Geometry: final body of the model. Coordinates: model frame, mm. A direction names the side the tool comes from. Give positions to 0.01 mm unless a question says otherwise; leave off trailing zeros. Order: outer loops, then holes, each group sorted by start corner. A loop starts at its lowest first (then second) coordinate and runs counter-clockwise, first axis right, second up. Notation, with made-up numbers: (-35, -31) -> (-23, -31) arc R10 cw to (-23, -24) -> close; hole circle Ø8 at (-31.75, 75). An arc over 180 degrees is marked (long way). Write item = value, one per line.
Solid Edge part; units mm, degrees
sketch "Sketch1" plane through (0, 0, 0) normal (0, -1, 0) x (1, 0, 0)
  line L0 (-60, 37) -> (-15, 0)
  line L1 (-15, 0) -> (15, 0)
  line L2 (15, 0) -> (60, 37)
  line L3 (60, 37) -> (-60, 37)
  dimension "D1" = 15
  dimension "D2" = 60
  dimension "D3" = 60
extrude "Protrusion1" add sketch "Sketch1" against normal blind 40
sketch "Sketch2" plane through (0, 40, 18.5) normal (0, 1, 0) x (-1, 0, 0)
  line L0 (-8, -18.5) -> (8, -18.5)
  line L1 (8, -18.5) -> (8, 11.5)
  line L2 (8, 11.5) -> (-8, 11.5)
  line L3 (-8, 11.5) -> (-8, -18.5)
  line L4 (-40.4647, 11.5) -> (-15, -9.4376)
  line L5 (-15, -9.4376) -> (-15, 11.5)
  line L6 (-15, 11.5) -> (-40.4647, 11.5)
  line L7 (40.4647, 11.5) -> (15, -9.4376)
  line L8 (15, -9.4376) -> (15, 11.5)
  line L9 (15, 11.5) -> (40.4647, 11.5)
  dimension "D1" = 8
extrude "ExtrudedCutout_1" cut sketch "Sketch2" against normal blind 33
sketch "Sketch3" plane through (0, 7, 15) normal (0, 1, 0) x (-1, 0, 0)
  circle A0 centre (0, -11.5) radius 1.7
  circle A1 centre (0, 4.5) radius 1.7
extrude "Cutout1" cut sketch "Sketch3" against normal through all
sketch "Sketch4" plane through (0, 0, 0) normal (1, 0, 0) x (0, 1, 0)
  line L0 (7, 0) -> (40, 30)
extrude "Cutout2" cut sketch "Sketch4" against normal through all and the other way through all material side at (0, 23.5336, 14.963)
sketch "Sketch5" plane through (0, 0, 0) normal (1, 0, 0) x (0, 1, 0)
  line L0 (40, 37) -> (40, 58)
  line L1 (40, 58) -> (33, 58)
  line L2 (33, 58) -> (33, 40)
  arc A0 (30, 37) -> (33, 40) centre (30, 40) ccw
  line L3 (40, 37) -> (30, 37)
  dimension "D1" = 40
  dimension "D2" = 40
extrude "ExtrudedProtrusion_3" add sketch "Sketch5" along normal mid plane 120
fillet "Round_1" radius 3 1 edges at (0, 0, 37)
extrude "Cutout3" [suppressed]
sketch "Sketch6" plane through (0, 33, 49) normal (0, -1, 0) x (1, 0, 0)
  line L0 (-50, 1.7) -> (50, 1.7)
  arc A0 (50, 1.7) -> (50, -1.7) centre (50, 0) cw
  line L1 (50, -1.7) -> (-50, -1.7)
  arc A1 (-50, 1.7) -> (-50, -1.7) centre (-50, 0) ccw
  dimension "D1" = 50
extrude "ExtrudedProtrusion_4" add sketch "Sketch6" along normal blind 25
properties material "ABS Plastic, medium impact"
1) Section query B-B (y = 13). Output: boundary loops of the cut face in (x, z).
Check sheet entries:
outline = (-60, 37) -> (-21.63, 5.45) -> (-8, 5.45) -> (-8, 30) -> (8, 30) -> (8, 5.45) -> (21.63, 5.45) -> (60, 37) -> close; (-50, 47.3) -> (50, 47.3) arc R1.7 ccw to (50, 50.7) -> (-50, 50.7) arc R1.7 ccw to start; hole (-40.46, 30) -> (-15, 9.06) -> (-15, 30) -> close; hole (15, 9.06) -> (40.46, 30) -> (15, 30) -> close
2) First-contact query: P1, Ø24, axis at y = 18.5, z = 10, coming from the -X side; P2, Ø6.5, axis at y = 24, z = 22.5, coming from the -X side; P3, Ø5.5, axis at x = -25.5, z = 48.5, coming from the -Y side; P4, Ø4, axis at x = 0, z = 3.5, coming from the -Y side. Flat tips, straight axial feed; report the tip coordinate or a pass-through.
Check sheet entries:
P1 = -41.76
P2 = -46.32
P3 = 8
P4 = 0
3) Mould query, pull axis X, two halves, no side actions, for faces 4 (the face through (1, 8, 49)), 5 (the face through (-51.7, 20.7, 49)), 6 (the face through (-15, 20, 22)). Classes: +X half, -X half, draft (parallel to the pull), parting line (faces both ways), or undercut.
Check sheet entries:
face_4 = draft
face_5 = -X half
face_6 = undercut
4) Section query A-A (x = 0). Output: boundary loops of the cut face in (y, z), plus the area to 3 significant figures.
Check sheet entries:
outline = (0, 0) -> (7, 0) -> (7, 1.8) -> (0, 1.8) -> close; (0, 5.2) -> (7, 5.2) -> (7, 17.8) -> (0, 17.8) -> close; (0, 21.2) -> (7, 21.2) -> (7, 30) -> (40, 30) -> (40, 58) -> (33, 58) -> (33, 50.7) -> (8, 50.7) -> (8, 47.3) -> (33, 47.3) -> (33, 40) arc R3 cw to (30, 37) -> (3, 37) arc R3 ccw to (0, 34) -> close
area = 674 mm²
5) Line query: line 1 (Z direction, x = 0, y = 5.25); line 2 (Z direction, x = 0, y = 1.5); line 3 (X direction, y = 12, z = 6.5). Output: solid intervals per line, ascending. Write a range as from..to.
Check sheet entries:
line_1 = 0..1.8, 5.2..17.8, 21.2..37
line_2 = 0..1.8, 5.2..17.8, 21.2..36.6
line_3 = -22.91..-8, 8..22.91
6) Section query C-C (z = 49). Output: boundary loops of the cut face in (x, y).
Check sheet entries:
outline = (-60, 33) -> (-51.7, 33) -> (-51.7, 8) -> (51.7, 8) -> (51.7, 33) -> (60, 33) -> (60, 40) -> (-60, 40) -> close
7) Reachability of faces 1 (the face through (-1, 21, 50.7)), 2 (the face through (8, 16, 22)), 3 (the face through (22, 7, 24)) from +Z, -Z, +X, -X, +Y, -Y: full face, straight path, thin tool, end or side. Return the list, or none.
Check sheet entries:
face_1 = +Z, +X, -X, -Y
face_2 = -Z, +Y
face_3 = +Y
8) Section query D-D (y = 23). Output: boundary loops of the cut face in (x, z), plus the area to 3 significant figures.
Check sheet entries:
outline = (-60, 37) -> (-32.69, 14.55) -> (-21.67, 14.55) -> (-40.46, 30) -> (-15, 30) -> (-15, 14.55) -> (-8, 14.55) -> (-8, 30) -> (8, 30) -> (8, 14.55) -> (15, 14.55) -> (15, 30) -> (40.46, 30) -> (21.67, 14.55) -> (32.69, 14.55) -> (60, 37) -> close; (-50, 47.3) -> (50, 47.3) arc R1.7 ccw to (50, 50.7) -> (-50, 50.7) arc R1.7 ccw to start
area = 1,690 mm²
